Work out the finished part from the listing and answer in its coordinate system (mm). Give positions to 0.01 mm unless a question says otherwise; leave off trailing zeros. Write each loop counter-clockwise with the first axis right and the second up, starting at its lowest first coordinate (ties: lowest second). Pieces come first, ordered by that corner, then holes.
1) Find section B-B (z = 1). Count the separate pieces of the cut face and the enclosed holes in it, plus the area to 3 significant figures.
2) Find section A-A (x = 0). Determine the outline of the cut face in (y, z), plus the area to 3 significant figures.
3) Given pin 1 Ø4 at (x, y) = (30.31, -17.5) entering from -Z, flat-ended and moving along its own axis, determine where the tip first touches the part or whether it passes through.
4) Find section D-D (x = 15.5). Determine the outline of the cut face in (y, z).
5) Find section C-C (y = -35). Determine the outline of the cut face in (x, z), plus the area to 3 significant figures.
6) Straight lines are drawn through the part: probe 1 along Y at (x, z) = (0, 3.95); probe 2 along Y at (x, z) = (15.5, 3.45); probe 3 along Y at (x, z) = (16, 3.45). For each, find the intervals that lie inside material, in ascending order.
Autodesk Inventor part; units mm, degrees
ref_plane "YZ Plane" through (0, 0, 0) normal (1, 0, 0) x (0, 1, 0)
ref_plane "XZ Plane" through (0, 0, 0) normal (0, 1, 0) x (-1, 0, 0)
ref_plane "XY Plane" through (0, 0, 0) normal (0, 0, 1) x (1, 0, 0)
sketch "Sketch1" plane through (0, 0, 0) normal (0, 0, 1) x (1, 0, 0)
  line L0 (-40, -40) -> (40, -40)
  line L1 (40, -40) -> (40, 40)
  line L2 (40, 40) -> (-40, 40)
  line L3 (-40, 40) -> (-40, -40)
  line L4 (-40, -40) -> (40, 40) construction
  line L5 (40, -40) -> (-40, 40) construction
  point P0 (0, 0)
  dimension "d0" = 80
  dimension "d1" = 80
extrude "Extrusion1" add sketch "Sketch1" along normal blind 5
sketch "Sketch2" plane through (0, 0, 5) normal (0, 0, 1) x (1, 0, 0)
  circle A0 centre (0, 0) radius 3
  circle A1 centre (0, 35) radius 2.5
  circle A2 centre (-30.3109, 17.5) radius 2.5
  circle A3 centre (-30.3109, -17.5) radius 2.5
  circle A4 centre (0, -35) radius 2.5
  circle A5 centre (30.3109, -17.5) radius 2.5
  circle A6 centre (30.3109, 17.5) radius 2.5
  line L0 (-15.5, -15.5) -> (15.5, -15.5) construction
  line L1 (15.5, -15.5) -> (15.5, 15.5) construction
  line L2 (15.5, 15.5) -> (-15.5, 15.5) construction
  line L3 (-15.5, 15.5) -> (-15.5, -15.5) construction
  line L4 (-15.5, -15.5) -> (15.5, 15.5) construction
  line L5 (15.5, -15.5) -> (-15.5, 15.5) construction
  circle A7 centre (-15.5, 15.5) radius 1.5
  circle A8 centre (15.5, 15.5) radius 1.5
  circle A9 centre (15.5, -15.5) radius 1.5
  circle A10 centre (-15.5, -15.5) radius 1.5
  dimension "d4" = 6
  dimension "d5" = 5
  dimension "d6" = 35
  dimension "d9" = 360
  dimension "d11" = 31
  dimension "d12" = 31
  dimension "d13" = 3
  dimension "d14" = 3
  dimension "d15" = 3
  dimension "d16" = 3
extrude "Extrusion2" cut sketch "Sketch2" against normal through all
properties part number "HA003" material "ABS Plastic"
Results:
1. separate pieces: 1
1. enclosed holes: 11
1. area: 6,230 mm2
2. outline: (-40, 0) - (-37.5, 0) - (-37.5, 5) - (-40, 5) - close; (-32.5, 0) - (-3, 0) - (-3, 5) - (-32.5, 5) - close; (3, 0) - (32.5, 0) - (32.5, 5) - (3, 5) - close; (37.5, 0) - (40, 0) - (40, 5) - (37.5, 5) - close
2. area: 320 mm2
3. pin 1: passes through
4. outline: (-40, 0) - (-17, 0) - (-17, 5) - (-40, 5) - close; (-14, 0) - (14, 0) - (14, 5) - (-14, 5) - close; (17, 0) - (40, 0) - (40, 5) - (17, 5) - close
5. outline: (-40, 0) - (-2.5, 0) - (-2.5, 5) - (-40, 5) - close; (2.5, 0) - (40, 0) - (40, 5) - (2.5, 5) - close
5. area: 375 mm2
6. probe 1: y = -40 to -37.5, -32.5 to -3, 3 to 32.5, 37.5 to 40
6. probe 2: y = -40 to -17, -14 to 14, 17 to 40
6. probe 3: y = -40 to -16.91, -14.09 to 14.09, 16.91 to 40
